Geometry check sheet. Reference: the model listing, model coordinates, mm. Round coordinates to 2 decimals unless told otherwise and drop trailing zeros. Order: outer loops, then holes, each group sorted by start corner. A loop starts at its lowest first (then second) coordinate and runs counter-clockwise, first axis right, second up. Notation, with made-up numbers: (-14, 23) - (7, 23) arc R31 cw to (7, 62) - close; hole circle Ø6 at (35, 35). An arc over 180 degrees is marked (long way). Return JSON: item names as keys, results as strings. Group by question number.
Q1. Sectioned sample at A-A, the plane x = -33. Record the cut outline in (y, z), then the cut area to 3 significant figures.
Q2. Sectioned sample at B-B, the plane y = -42.5. Give the number of separate pieces and of enclosed holes in the cut face, then the cut area to 3 significant figures.
Q3. Gauge pin test, flat ends, axial feed: pin 1 Ø12 at (y, z) = (-43.5, 21.5) entering from -X; pin 2 Ø8 at (x, y) = (36.5, -27.5) entering from +Z; pin 3 Ø10 at (x, y) = (35, -43) entering from +Z. Record the tip position at first contact, or that the pin passes through.
Q4. Sectioned sample at C-C, the plane z = 6.5. Record the cut outline in (x, y).
Q5. Sectioned sample at D-D, the plane x = -17. Record the cut outline in (y, z), then the cut area to 3 significant figures.
Q6. Material ranges on line 1 along X through (y, z) = (-14.5, 1); line 2 along Z through (x, y) = (38.5, -3); line 3 along Z through (x, y) = (38, -8), recorded low to high.
```python
from build123d import *

# Parameters (mm, degrees)
F2_DEPTH = 50.8
F3_D     = 6.35


with BuildPart() as f2:
    # F0 (on Front) → F2 (new body)
    with BuildSketch(Plane.XZ):
        with BuildLine():
            ThreePointArc((-21.131788, -23.46847), (-11.433926, -13.47147), (-7.897254, 0))
            ThreePointArc((-7.897254, 0), (-12.99061, 15.919526), (-26.378829, 25.925983))
            ThreePointArc((-26.378829, 25.925983), (-62.594401, -2.897016), (-21.131788, -23.46847))
        make_face()
        with BuildLine():
            ThreePointArc((-26.378829, 25.925983), (-12.99061, 15.919526), (-7.897254, 0))
            ThreePointArc((-7.897254, 0), (-11.433926, -13.47147), (-21.131788, -23.46847))
            Line((-21.131788, -23.46847), (40.957866, -16.070068))
            ThreePointArc((40.957866, -16.070068), (22.860697, 0.215672), (41.385461, 16.013328))
            Line((41.385461, 16.013328), (-26.378829, 25.925983))
        make_face()
        with BuildLine():
            ThreePointArc((55.226759, 0), (51.286853, 10.583102), (41.385461, 16.013328))
            ThreePointArc((41.385461, 16.013328), (22.860697, 0.215672), (40.957866, -16.070068))
            ThreePointArc((40.957866, -16.070068), (51.144731, -10.745329), (55.226759, 0))
        make_face()
    extrude(amount=F2_DEPTH)

    # F3 (through all)
    with Locations(Plane(origin=(0, 0, 0), x_dir=(1, 0, 0), z_dir=(0, 1, 0))):
        with Locations((-34.853246, 0), (39.460354, 0)):
            Hole(F3_D / 2)


solid = f2.part
```
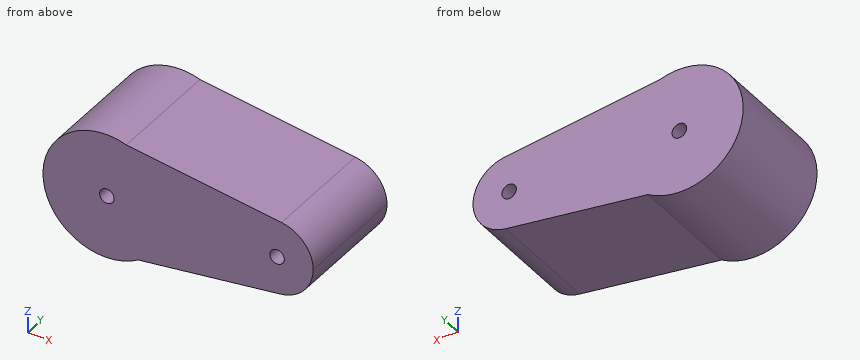
Reply:
{
 "1": {"outline": "(-50.8, -27.33) - (0, -27.33) - (0, -2.58) - (-50.8, -2.58) - close; (-50.8, 2.58) - (0, 2.58) - (0, 27.33) - (-50.8, 27.33) - close", "area": "2,510 mm^2"},
 "2": {"separate pieces": "1", "enclosed holes": "2", "area": "4,720 mm^2"},
 "3": {"pin 1": "x = -57.95", "pin 2": "z = 17.31", "pin 3": "z = 17.68"},
 "4": {"outline": "(-61.97, -50.8) - (53.86, -50.8) - (53.86, 0) - (-61.97, 0) - close"},
 "5": {"outline": "(-50.8, -22.98) - (0, -22.98) - (0, 24.55) - (-50.8, 24.55) - close", "area": "2,410 mm^2"},
 "6": {"line 1": "-62.73 to -37.87, -31.84 to 36.45, 42.47 to 55.2", "line 2": "-16.36 to -3.03, 3.03 to 16.44", "line 3": "-16.42 to -2.82, 2.82 to 16.51"}
}
